Design review of the part built by this model. Coordinates are the model's own, in mm. A direction names the side the tool comes from. Coordinates: 2 decimals unless noted, no trailing zeros. Loops run counter-clockwise (first coordinate to the right, second up) from the corner with the lowest first, then second, coordinate; pieces in that order, holes last. Notation, with made-up numbers: (84.5, 56) -> (119.5, 56) arc R8 cw to (119.5, 60) -> close; hole circle Ø2 at (32, 19.5). An arc over 180 degrees is marked (long way). Answer as a JSON object with one key per item and string values.
```python
from build123d import *

# Parameters (mm, degrees)
F0_R     = 4.4958
F0_R_2   = 1.5875
F1_DEPTH = 6.35
F2_R     = 12.7
F2_R_2   = 1.7526
F2_R_3   = 1.5875
F3_DEPTH = 2.54
F4_W     = 0.254
F4_H     = 2.54
F5_DEPTH = 25.4


with BuildPart() as f1:
    # F0 (on Top) → F1 (new body)
    with BuildSketch(Plane.XY):
        Circle(F0_R)
        Circle(F0_R_2, mode=Mode.SUBTRACT)
    extrude(amount=F1_DEPTH)

    # F2 (on face) → F3 (join)
    with BuildSketch(Plane.XY.offset(6.35)):
        Circle(F2_R)
        with Locations((0, -9.6901)):
            Circle(F2_R_2, mode=Mode.SUBTRACT)
        with Locations((-8.3918727652, -4.84505)):
            Circle(F2_R_2, mode=Mode.SUBTRACT)
        Circle(F2_R_3, mode=Mode.SUBTRACT)
        with Locations((8.3918727652, -4.84505)):
            Circle(F2_R_2, mode=Mode.SUBTRACT)
        with Locations((-8.3918727652, 4.84505)):
            Circle(F2_R_2, mode=Mode.SUBTRACT)
        with Locations((0, 9.6901)):
            Circle(F2_R_2, mode=Mode.SUBTRACT)
        with Locations((8.3918727652, 4.84505)):
            Circle(F2_R_2, mode=Mode.SUBTRACT)
    extrude(amount=F3_DEPTH)

    # F4 (on face) → F5 (cut)
    with BuildSketch(Plane.XY.offset(8.89)):
        with BuildLine():
            Line((-4.2418, 0), (-4.4958, 0))
            ThreePointArc((-4.4958, 0), (-4.2552090791, -1.45100425), (-3.5591865681, -2.7467086874))
            Line((-3.5591865681, -2.7467086874), (-3.3648710152, -2.5827331048))
            ThreePointArc((-3.3648710152, -2.5827331048), (-4.0165891695, -1.3637736923), (-4.2418, 0))
        make_face()
        with Locations((4.3688, 8.3054968122)):
            Rectangle(F4_W, F4_H)
        with Locations((4.3688, 5.1822738967)):
            Rectangle(F4_W, F4_H)
        with BuildLine():
            ThreePointArc((2.3889624864, -3.5050999242), (-0.0460958584, -4.2415495296), (-2.4645739513, -3.4523531799))
            Line((-2.4645739513, -3.4523531799), (-2.6152441527, -3.656872388))
            ThreePointArc((-2.6152441527, -3.656872388), (-0.0391240272, -4.4956297613), (2.5512036829, -3.7018343302))
            Line((2.5512036829, -3.7018343302), (2.3889624864, -3.5050999242))
        make_face()
        with Locations((-4.3688, 8.3054968122)):
            Rectangle(F4_W, F4_H)
        with Locations((-4.3688, 5.1822738967)):
            Rectangle(F4_W, F4_H)
        with Locations((-4.3688, 2.0590509812)):
            Rectangle(F4_W, F4_H)
        with Locations((4.3688, 2.0590509812)):
            Rectangle(F4_W, F4_H)
        with BuildLine():
            ThreePointArc((3.7276640074, -2.5133122941), (4.2994795897, -1.3140368708), (4.4958, 0))
            Line((4.4958, 0), (4.2418, 0))
            ThreePointArc((4.2418, 0), (4.0608262018, -1.2257886437), (3.5333470796, -2.3469822444))
            Line((3.5333470796, -2.3469822444), (3.7276640074, -2.5133122941))
        make_face()
        Polygon((-4.4958, 11.8806733481), (-4.4958, 10.3643210605), (-4.2418, 10.3643210605), (-4.2418, 11.9706780409), align=None)
        Polygon((4.2418, 11.973758473), (4.2418, 10.3643210605), (4.4958, 10.3643210605), (4.4958, 11.8776168637), align=None)
    extrude(amount=-F5_DEPTH, mode=Mode.SUBTRACT)


solid = f1.part
```
1) Wall thickness on probe 1 along Y at (x, z) = (0, 3.25); probe 2 along Z at (x, y) = (4.25, 6.5); probe 3 along X at (y, z) = (-4.75, 8.75): over which ranges is each line inside the solid? List them lowest first.
Completed:
{"probe 1": "-4.24 to -1.59, 1.59 to 4.5", "probe 2": "6.35 to 8.89", "probe 3": "-11.78 to -10.14, -6.64 to 6.64, 10.14 to 11.78"}
2) Clearance check with flat-ended pins moving along their axes: pin 1 Ø1 at (x, z) = (-3, 2.5) entering from -Y; pin 2 Ø2 at (y, z) = (5.5, 8) entering from +X; pin 3 Ø5.5 at (x, y) = (0, 9.69) entering from -Z. State where each tip first meets the part, or that it passes through.
Completed:
{"pin 1": "y = -3.66", "pin 2": "x = 11.88", "pin 3": "z = 6.35"}
3) Add section D-D, the plane x = 5. Give the boundary of the cut face in (y, z), and give its area (3 significant figures).
Completed:
{"outline": "(-11.67, 6.35) -> (11.67, 6.35) -> (11.67, 8.89) -> (-11.67, 8.89) -> close", "area": "59.3 mm²"}
4) Add section A-A, the plane x = 0. Give the boundary of the cut face in (y, z), and give its area (3 significant figures).
Completed:
{"outline": "(-12.7, 6.35) -> (-11.44, 6.35) -> (-11.44, 8.89) -> (-12.7, 8.89) -> close; (-7.94, 6.35) -> (-4.5, 6.35) -> (-4.5, 8.89) -> (-7.94, 8.89) -> close; (-4.24, 0) -> (-1.59, 0) -> (-1.59, 8.89) -> (-4.24, 8.89) -> close; (1.59, 0) -> (4.5, 0) -> (4.5, 6.35) -> (7.94, 6.35) -> (7.94, 8.89) -> (1.59, 8.89) -> close; (11.44, 6.35) -> (12.7, 6.35) -> (12.7, 8.89) -> (11.44, 8.89) -> close", "area": "73.3 mm²"}
5) For faces 1 (the flat face through (-4.242, 1, 5)), 2 (the cylindrical face through (0.078, 4.495, 3.131)), 3 (the flat face through (3, 0, 8.89)), list the 3-axis set-ups (+Z, -Z, +X, -X, +Y, -Y) from which the entire face can be reached by the end or side of a thin tool; tool diameter is ignored.
Completed:
{"face 1": "+Z, -Z", "face 2": "-Z, +Y", "face 3": "+Z, +X, -X, +Y, -Y"}
6) Add section C-C, the plane x = -6. Give the boundary of the cut face in (y, z).
Completed:
{"outline": "(-11.19, 6.35) -> (11.19, 6.35) -> (11.19, 8.89) -> (-11.19, 8.89) -> close"}
7) The part is to be moulded in two halves that separate along X. For faces 4 (the cylindrical face through (-10.143, 4.922, 7.602)), 5 (the cylindrical face through (0.1, 12.7, 7.6)), 6 (the flat face through (5, 0, 6.35)), say which applies: pulls with the +X half, pulls with the -X half, needs draft (parallel to the pull), parting line crosses it, or undercut.
Completed:
{"face 4": "undercut", "face 5": "parting line crosses it", "face 6": "needs draft"}
